```python
from build123d import *

# Parameters (mm, degrees)
SKETCH_2_R      = 1.65
SKETCH_2_R_2    = 2
EXTRUDE_1_DEPTH = 8
FILLET_1_R      = 3
FILLET_2_R      = 1


with BuildPart() as part:
    # 草图2 → 凸台-拉伸1 (new body)
    with BuildSketch(Plane.XY):
        Polygon((0, 18.963672443), (7.484579775, 12.963672443), (16.423022085, 9.481836222), (14.96915955, 0), (16.423022085, -9.481836222), (7.484579775, -12.963672443), (0, -18.963672443), (-7.484579775, -12.963672443), (-16.423022085, -9.481836222), (-14.96915955, 0), (-16.423022085, 9.481836222), (-7.484579775, 12.963672443), align=None)
        with Locations((0, 13.5)):
            Circle(SKETCH_2_R, mode=Mode.SUBTRACT)
        with Locations((11.691342951, 6.75)):
            Circle(SKETCH_2_R, mode=Mode.SUBTRACT)
        with Locations((11.691342951, -6.75)):
            Circle(SKETCH_2_R, mode=Mode.SUBTRACT)
        with Locations((0, -13.5)):
            Circle(SKETCH_2_R, mode=Mode.SUBTRACT)
        with Locations((-11.691342951, -6.75)):
            Circle(SKETCH_2_R, mode=Mode.SUBTRACT)
        with Locations((-11.691342951, 6.75)):
            Circle(SKETCH_2_R, mode=Mode.SUBTRACT)
        with Locations((6, 10.392304845)):
            Circle(SKETCH_2_R_2, mode=Mode.SUBTRACT)
        with Locations((12, 0)):
            Circle(SKETCH_2_R_2, mode=Mode.SUBTRACT)
        with Locations((6, -10.392304845)):
            Circle(SKETCH_2_R_2, mode=Mode.SUBTRACT)
        with Locations((-6, -10.392304845)):
            Circle(SKETCH_2_R_2, mode=Mode.SUBTRACT)
        with Locations((-12, 0)):
            Circle(SKETCH_2_R_2, mode=Mode.SUBTRACT)
        with Locations((-6, 10.392304845)):
            Circle(SKETCH_2_R_2, mode=Mode.SUBTRACT)
        with BuildLine():
            Line((0, -7.5), (2, -7.5))
            Line((2, -7.5), (2, -5.656854249))
            ThreePointArc((2, -5.656854249), (0, 6), (-2, -5.656854249))
            Line((-2, -5.656854249), (-2, -7.5))
            Line((-2, -7.5), (0, -7.5))
        make_face(mode=Mode.SUBTRACT)
    extrude(amount=EXTRUDE_1_DEPTH)

    # 圆角1
    fillet_1_edges = [part.edges().sort_by_distance(p)[0] for p in [
        (0, 18.963672443, 4),
        (7.484579775, 12.963672443, 4),
        (16.423022085, 9.481836222, 4),
        (14.96915955, 0, 4),
        (16.423022085, -9.481836222, 4),
        (7.484579775, -12.963672443, 4),
        (0, -18.963672443, 4),
        (-7.484579775, -12.963672443, 4),
        (-16.423022085, -9.481836222, 4),
        (-14.96915955, 0, 4),
        (-16.423022085, 9.481836222, 4),
        (-7.484579775, 12.963672443, 4),
    ]]
    fillet(fillet_1_edges, radius=FILLET_1_R)

    # 圆角2
    fillet_2_edges = [part.edges().sort_by_distance(p)[0] for p in [
        (-2, -7.5, 4),
        (2, -7.5, 4),
        (2, -5.656854249, 4),
        (-2, -5.656854249, 4),
    ]]
    fillet(fillet_2_edges, radius=FILLET_2_R)


solid = part.part
```
Read the model definition and answer for the solid it produces. Units are mm, in the model's axes. A direction names the side the tool comes from. Give positions to 0.01 mm unless a question says otherwise; leave off trailing zeros. Loops run counter-clockwise (first coordinate to the right, second up) from the corner with the lowest first, then second, coordinate; pieces in that order, holes last.
Item 1: For faces 1 (the flat face through (11.004, 11.593, 3.944)), 2 (the cylindrical face through (2.16, -5.78, 4.06)), determine the directions among +Z, -Z, +X, -X, +Y, -Y from which every point of the face is accessible in a straight line to the end or side of a thin tool.
Item 2: The part is cut by section B-B (x = 0). Write down the section's boundary in (y, z).
Item 3: The part is cut by section D-D (x = 9). Write down the section's boundary in (y, z), and give its area (3 significant figures).
Item 4: The mould has two halves that part along Y. Classify faces 3 (the flat face through (4.538, -15.326, 3.944)), 4 (the flat face through (15.54, -3.73, 3.94)), 5 (the flat face through (7, 0, 0)), 6 (the flat face through (-11.09, 11.56, 3.94)): released by +Y, released by -Y, zero draft, split by the parting line, or undercut.
Item 5: Find the intervals of material crossed by line 1 along Y through (x, z) = (-12, 2); line 2 along X through (y, z) = (10, 1); line 3 along X through (y, z) = (1, 3.5), in increasing order.
Item 6: The part is cut by section C-C (z = 5). Give the number of separate pieces and of enclosed holes in the cut face, and give its area (3 significant figures).
Item 7: Each of these flat-tipped pins is pushed along its axis until it touches: pin 1 Ø2 at (y, z) = (9.5, 5.5) entering from -X; pin 2 Ø2.5 at (x, y) = (6, -10.39) entering from +Z. Where does it stop, or does it pass through?
Item 8: The part is cut by section A-A (y = 0). Write down the section's boundary in (x, z).
Taken from the geometry:
1. face 1: +Z, -Z, +X, +Y
1. face 2: +Z, -Z
2. outline: (-18.12, 0) - (-15.15, 0) - (-15.15, 8) - (-18.12, 8) - close; (-11.85, 0) - (-7.5, 0) - (-7.5, 8) - (-11.85, 8) - close; (6, 0) - (11.85, 0) - (11.85, 8) - (6, 8) - close; (15.15, 0) - (18.12, 0) - (18.12, 8) - (15.15, 8) - close
3. outline: (-12.37, 0) - (12.37, 0) - (12.37, 8) - (-12.37, 8) - close
3. area: 198 mm2
4. face 3: released by -Y
4. face 4: undercut
4. face 5: zero draft
4. face 6: released by +Y
5. line 1: y = -11.2 to -8.37, -5.13 to -2, 2 to 5.13, 8.37 to 11.2
5. line 2: x = -14.84 to -7.96, -4.04 to 4.04, 7.96 to 14.84
5. line 3: x = -15.12 to -13.73, -10.27 to -5.92, 5.92 to 10.27, 13.73 to 15.12
6. separate pieces: 1
6. enclosed holes: 13
6. area: 599 mm2
7. pin 1: stops at x = -15.94
7. pin 2: passes through
8. outline: (-15, 0) - (-14, 0) - (-14, 8) - (-15, 8) - close; (-10, 0) - (-6, 0) - (-6, 8) - (-10, 8) - close; (6, 0) - (10, 0) - (10, 8) - (6, 8) - close; (14, 0) - (15, 0) - (15, 8) - (14, 8) - close
